Source: CAD feature listing. Evaluate the final solid. Frame: model axes, mm. Round coordinates to 2 decimals unless told otherwise and drop trailing zeros. Loops run counter-clockwise (first coordinate to the right, second up) from the corner with the lowest first, then second, coordinate; pieces in that order, holes last. Notation, with made-up numbers: M 72,74.5 L 105,74.5 A17 cw 105,95.5 Z; hole C -37,54.25 d1. An arc over 180 degrees is marked long. Answer as a JSON object with one key per item and string values.
Autodesk Inventor part; units mm, degrees
ref_plane "YZ Plane" through (0, 0, 0) normal (1, 0, 0) x (0, 1, 0)
ref_plane "XZ Plane" through (0, 0, 0) normal (0, 1, 0) x (-1, 0, 0)
ref_plane "XY Plane" through (0, 0, 0) normal (0, 0, 1) x (1, 0, 0)
sketch "스케치1" plane through (0, 0, 0) normal (0, 0, 1) x (1, 0, 0)
  line L0 (-13.75, 0) -> (13.75, 0)
  line L1 (-8.15, 0) -> (-4.075, 7.0581)
  line L2 (-4.075, 7.0581) -> (4.075, 7.0581)
  line L3 (4.075, 7.0581) -> (8.15, 0)
  line L4 (8.15, 0) -> (4.075, -7.0581)
  line L5 (4.075, -7.0581) -> (-4.075, -7.0581)
  line L6 (-4.075, -7.0581) -> (-8.15, 0)
  line L7 (-5.8071, 10.0581) -> (-11.6141, 0)
  line L8 (-11.6141, 0) -> (-5.8071, -10.0581)
  line L9 (-5.8071, -10.0581) -> (5.8071, -10.0581)
  line L10 (5.8071, -10.0581) -> (11.6141, 0)
  line L11 (11.6141, 0) -> (5.8071, 10.0581)
  line L12 (5.8071, 10.0581) -> (-5.8071, 10.0581)
  line L13 (-13.75, 0) -> (-13.75, 3)
  line L14 (-13.75, 3) -> (-9.8821, 3)
  line L15 (13.75, 0) -> (13.75, 3)
  line L16 (13.75, 3) -> (9.8821, 3)
  point P0 (0, 0)
  point P1 (0, 0)
  point P2 (0, 0)
  point P3 (8.15, 0)
  dimension "d0" = 27.5
  dimension "d1" = 16.3
  dimension "d2" = 3
  dimension "d3" = 3
  dimension "d4" = 3
extrude "돌출1" add sketch "스케치1" along normal mid plane 4 contours L13 L14 L7 L0 | L7 L12 L11 L0 L3 L2 L1 | L11 L16 L15 L0
sketch "스케치2" plane through (-13.75, 3, 2) normal (0, 1, 0) x (1, 0, 0)
  line L0 (1.75, -6.7825) -> (25.75, -6.7825)
  line L1 (25.75, -6.7825) -> (25.75, 6.7825) construction
  line L2 (25.75, 6.7825) -> (1.75, 6.7825)
  line L3 (1.75, 6.7825) -> (1.75, -6.7825) construction
  line L4 (9.675, 0) -> (17.825, 0)
  line L5 (1.75, -6.7825) -> (25.75, 6.7825) construction
  line L6 (25.75, -6.7825) -> (1.75, 6.7825) construction
  circle A0 centre (1.75, 2) radius 1.15
  circle A1 centre (25.75, 2) radius 1.15
  line L7 (0, 4) -> (3.8679, 4)
  point P0 (13.75, 2)
  point P1 (13.75, 0)
  dimension "d7" = 24
  dimension "d8" = 2.3
  dimension "d9" = 2.3
  dimension "d10" = 2
extrude "돌출2" cut sketch "스케치2" against normal blind 4
properties part number "카스벨브 하단 커버"
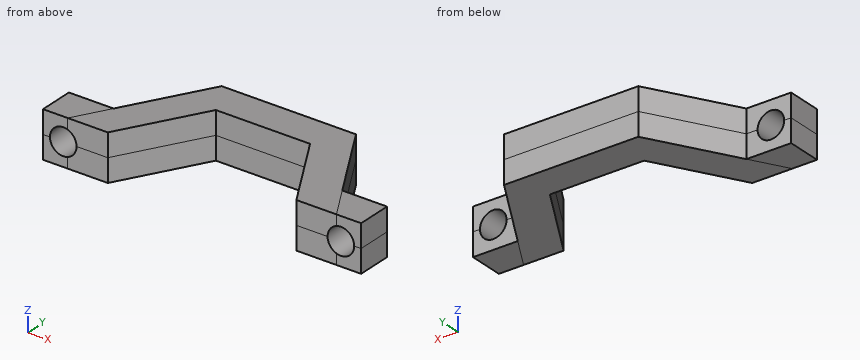
Item 1: Section D-D on y = 5.5. Return the cut outline in (x, z).
Answer sheet:
{"outline": "M -8.44,-2 L -4.97,-2 L -4.97,2 L -8.44,2 Z; M 4.97,-2 L 8.44,-2 L 8.44,2 L 4.97,2 Z"}
Item 2: Section B-B on x = 12. Return the cut outline in (y, z), then the cut area to 3 significant figures.
Answer sheet:
{"outline": "M 0,-2 L 3,-2 L 3,-1.15 L 0,-1.15 Z; M 0,1.15 L 3,1.15 L 3,2 L 0,2 Z", "area": "5.10 mm²"}
Item 3: Section C-C on z = 1.65. Return the cut outline in (x, y) (3 decimals), then the cut area to 3 significant figures.
Answer sheet:
{"outline": "M -13.75,0 L -8.15,0 L -4.075,7.058 L 4.075,7.058 L 8.15,0 L 13.75,0 L 13.75,3 L 9.882,3 L 5.807,10.058 L -5.807,10.058 L -9.882,3 L -13.75,3 Z", "area": "107 mm²"}
Item 4: Line query: probe 1 along Z at (x, y) = (-12, 1.9); probe 2 along X at (y, z) = (1.7, 0); probe 3 along X at (y, z) = (1.5, 1). Output: solid intervals per line, ascending. Write a range as from..to.
Answer sheet:
{"probe 1": "z = -2..-1.15, 1.15..2", "probe 2": "x = -13.75..-13.15, -10.85..-7.17, 7.17..10.85, 13.15..13.75", "probe 3": "x = -13.75..-12.57, -11.43..-7.28, 7.28..11.43, 12.57..13.75"}
Item 5: Contact query for flat-ended pins moving along their axis: pin 1 Ø1.6 at (x, z) = (-12.5, -1) entering from +Y; pin 2 Ø0.6 at (x, z) = (2, -0.5) entering from -Y. Output: stop coordinate, or through.
Answer sheet:
{"pin 1": "stops at y = 3", "pin 2": "stops at y = 7.06"}
Item 6: Section A-A on y = 1.25. Return the cut outline in (x, z), then the cut area to 3 significant figures.
Answer sheet:
{"outline": "M -13.75,-2 L -7.43,-2 L -7.43,2 L -13.75,2 Z; M 7.43,-2 L 13.75,-2 L 13.75,2 L 7.43,2 Z; hole C -12,0 d2.3; hole C 12,0 d2.3", "area": "42.3 mm²"}
